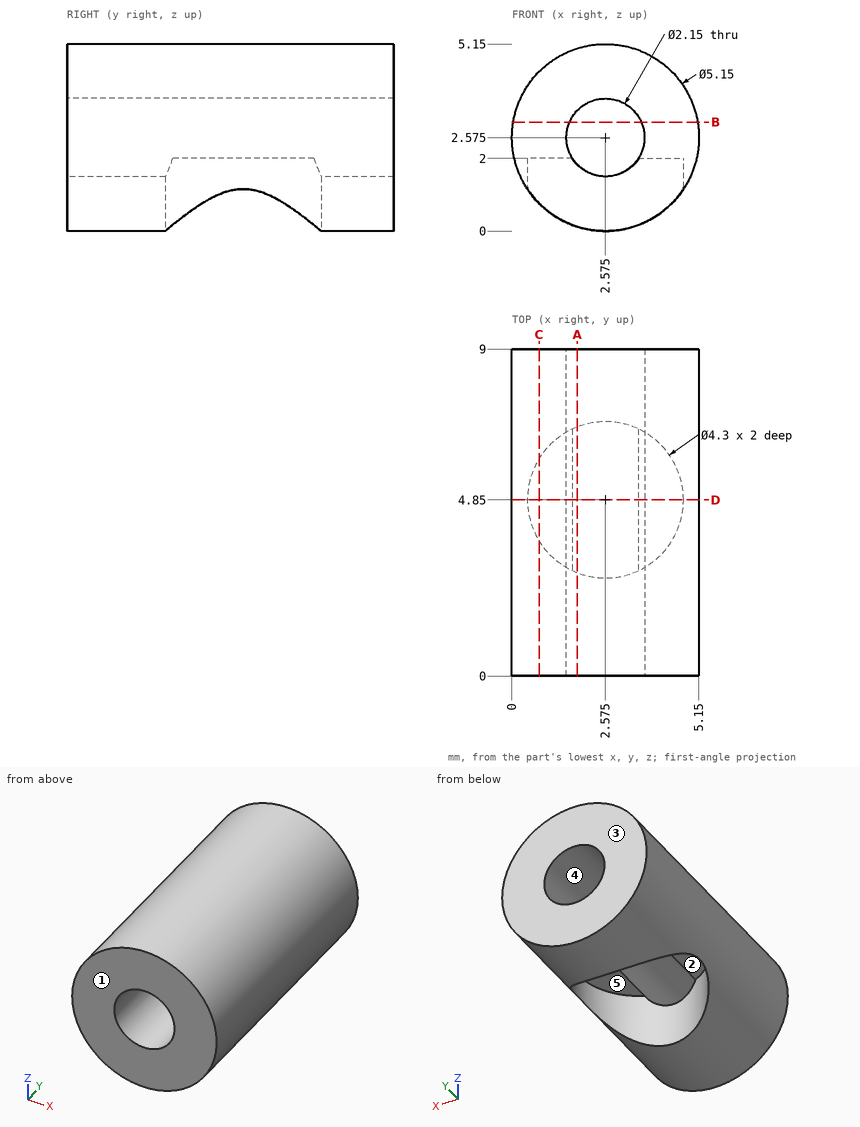
Input: dimensioned drawing with shaded views. Units: mm. Origin: part minimum x, y, z. A direction names the side the tool comes from. Round coordinates to 2 decimals unless told otherwise and drop trailing zeros. Order: outer loops, then holes, each group sorted by start corner. A loop starts at its lowest first (then second) coordinate and runs counter-clockwise, first axis right, second up. Notation, with made-up numbers: (28.25, 53) -> (80.25, 53) arc R20 cw to (80.25, 70) -> close; hole circle Ø8 at (-13, 88.5). An arc over 180 degrees is marked (long way). One line per item, written item: value. Start each with the question number.
Q1. Pin query (flat end, axial travel): pin 1 (1.5 mm diameter, centred on y = 4, z = 4, fed in from +X); pin 2 (1.4 mm diameter, centred on x = 4, y = 5.5, fed in from -Z). Return the tip coordinate at first contact, or that it passes through.
Q2. Section query C-C (x = 0.75). Return the cut outline in (y, z).
Q3. Material intervals for probe 1 along X at (y, z) = (7, 3.25); probe 2 along Y at (x, z) = (2.35, 0.95); probe 3 along Y at (x, z) = (1.2, 0.6), sorted ascending.
Q4. Section query D-D (y = 4.85). Return the cut outline in (x, z) (3 decimals), plus the area to 3 significant figures.
Q5. Access query for the marked faces 1 and 2. Directions: +Z, -Z, +X, -X, +Y, -Y. A direction counts if a zero-diameter tool reaches every point of the face in a straight line with its end or side. Return the directions, or none.
Q6. Section query A-A (x = 1.8). Return the cut outline in (y, z), plus the area to 3 significant figures.
Q7. Draft query along Y for the marked faces 3, 4 and 5. Return one class per face: pulls with the +Y half, pulls with the -Y half, needs draft (parallel to the pull), parting line crosses it, or undercut.
Q8. Section query B-B (z = 3). Return the cut outline in (x, y), plus the area to 3 significant figures.
Findings below:
1. pin 1: x = 5.06
1. pin 2: z = 0.66
2. outline: (0, 0.76) -> (3.71, 0.76) -> (3.71, 2) -> (5.99, 2) -> (5.99, 0.76) -> (9, 0.76) -> (9, 4.39) -> (0, 4.39) -> close
3. probe 1: 0.09 to 1.74, 3.41 to 5.06
3. probe 2: 0 to 2.71, 6.99 to 9
3. probe 3: 0 to 3.2, 6.5 to 9
4. outline: (0.425, 1.158) -> (0.425, 2) -> (1.667, 2) arc R1.075 cw (long way) to (3.483, 2) -> (4.725, 2) -> (4.725, 1.158) arc R2.575 ccw (long way) to start
4. area: 10.7 mm²
5. face 1: +Z, -Z, +X, -X, -Y
5. face 2: -Z
6. outline: (0, 0.12) -> (2.84, 0.12) -> (2.84, 1.83) -> (0, 1.83) -> close; (0, 3.32) -> (9, 3.32) -> (9, 5.03) -> (0, 5.03) -> close; (6.86, 0.12) -> (9, 0.12) -> (9, 1.83) -> (6.86, 1.83) -> close
6. area: 23.9 mm²
7. face 3: pulls with the +Y half
7. face 4: needs draft
7. face 5: undercut
8. outline: (0.04, 0) -> (1.59, 0) -> (1.59, 9) -> (0.04, 9) -> close; (3.56, 0) -> (5.11, 0) -> (5.11, 9) -> (3.56, 9) -> close
8. area: 27.9 mm²
